```python
from build123d import *

# Parameters (mm, degrees)
F0_W     = 76.2
F0_H     = 50.8
F0_R     = 12.7
F1_DEPTH = 25.4
F2_W     = 6.35
F2_H     = 50.8
F3_DEPTH = 2.54
F5_R     = 10.0587183536
F6_DEPTH = 25.4
F7_DEPTH = 12.446
F8_DEPTH = 70.358


with BuildPart() as f1:
    # F0 (on Top) → F1 (new body)
    with BuildSketch(Plane.XY):
        with Locations((3.2262094319, -2.200336157)):
            Rectangle(F0_W, F0_H)
        Circle(F0_R, mode=Mode.SUBTRACT)
    extrude(amount=F1_DEPTH)

    # F2 (on face) → F3 (cut)
    with BuildSketch(Plane.XY.offset(25.4)):
        with Locations((-29.1587905681, -2.200336157)):
            Rectangle(F2_W, F2_H)
        with BuildLine():
            Line((-6.35, -10.9985226281), (-6.35, -27.600336157))
            Line((-6.35, -27.600336157), (6.35, -27.600336157))
            Line((6.35, -27.600336157), (6.35, -10.9985226281))
            ThreePointArc((6.35, -10.9985226281), (0, -12.7), (-6.35, -10.9985226281))
        make_face()
        with BuildLine():
            Line((6.35, 23.199663843), (-6.35, 23.199663843))
            Line((-6.35, 23.199663843), (-6.35, 10.9985226281))
            ThreePointArc((-6.35, 10.9985226281), (0, 12.7), (6.35, 10.9985226281))
            Line((6.35, 10.9985226281), (6.35, 23.199663843))
        make_face()
    extrude(amount=-F3_DEPTH, mode=Mode.SUBTRACT)

    # F5 (on face) → F6 (join)
    with BuildSketch(Plane.YZ.offset(41.3262094319)):
        with Locations((-2.200336157, 12.7)):
            Circle(F5_R)
    extrude(amount=F6_DEPTH)

    # F5 (on face) → F7 (join)
    with BuildSketch(Plane.YZ.offset(41.3262094319)):
        with Locations((-2.200336157, 12.7)):
            Circle(F5_R)
    extrude(amount=-F7_DEPTH)

    # F4 (on face) → F8 (cut)
    with BuildSketch(Plane.XZ.offset(27.600336157)):
        Polygon((30.2859525938, 25.4), (17.5859525938, 25.4), (14.6530132263, 20.32), (33.2188919613, 20.32), align=None)
    extrude(amount=-F8_DEPTH, mode=Mode.SUBTRACT)


solid = f1.part
```
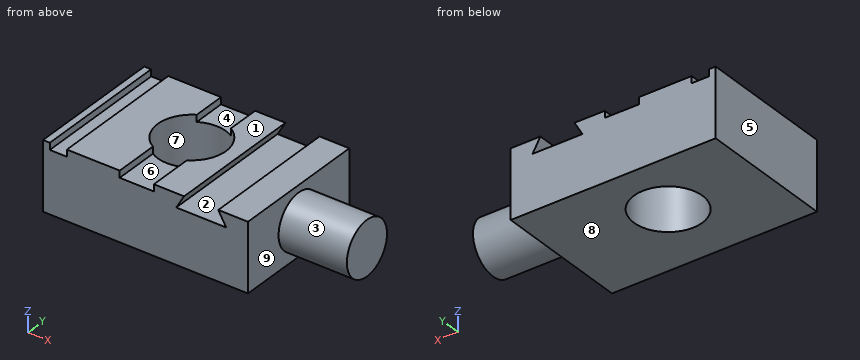
Read the model definition and answer for the solid it produces. Units are mm, in the model's axes. Face numbers are marked on the shaded views. A direction names the side the tool comes from. Give positions to 0.01 mm unless a question says otherwise; leave off trailing zeros. Order: outer loops, then holes, each group sorted by start corner. A loop starts at its lowest first (then second) coordinate and runs counter-clockwise, first axis right, second up. Notation, with made-up numbers: (77, -7) -> (129, -7) arc R18 ccw to (129, 19) -> close; hole circle Ø2 at (62.25, 43.5). An arc over 180 degrees is marked (long way). Write item = value, one per line.
1. A cutting plane is placed at A-A, the plane z = 21.75. Write down the section's boundary in (x, y), and give its area (3 significant figures).
Numbers:
outline = (-34.87, -27.6) -> (15.48, -27.6) -> (15.48, 23.2) -> (-34.87, 23.2) -> close; (32.39, -27.6) -> (41.33, -27.6) -> (41.33, -6.59) -> (66.73, -6.59) -> (66.73, 2.19) -> (41.33, 2.19) -> (41.33, 23.2) -> (32.39, 23.2) -> close; hole circle Ø25.4 at (0, 0)
area = 2,730 mm²
2. Given pin 1 (0.8 mm diameter, centred on y = 4.5, z = 24, fed in from +X); pin 2 (20.5 mm diameter, centred on x = 0, y = 0, fed in from -Z), each flat-ended and moving along its own axis, determine where each tip first touches the part or whether it passes through.
Numbers:
pin_1 = 41.33
pin_2 = through
3. A cutting plane is placed at B-B, the plane x = 0. Write down the section's boundary in (y, z), and give its area (3 significant figures).
Numbers:
outline = (-27.6, 0) -> (-12.7, 0) -> (-12.7, 22.86) -> (-27.6, 22.86) -> close; (12.7, 0) -> (23.2, 0) -> (23.2, 22.86) -> (12.7, 22.86) -> close
area = 581 mm²
4. Straight lines are drawn through the part: line 1 along Y through (x, z) = (0, 15.75); line 2 along X through (y, z) = (0, 18); line 3 along X through (y, z) = (0.5, 21.25). For each, find the intervals that lie inside material, in ascending order.
Numbers:
line_1 = -27.6 to -12.7, 12.7 to 23.2
line_2 = -34.87 to -12.7, 12.7 to 66.73
line_3 = -34.87 to -12.69, 12.69 to 15.19, 32.68 to 66.73
5. A cutting plane is placed at D-D, the plane z = 12.7. Write down the section's boundary in (x, y), and give its area (3 significant figures).
Numbers:
outline = (-34.87, -27.6) -> (41.33, -27.6) -> (41.33, -12.26) -> (66.73, -12.26) -> (66.73, 7.86) -> (41.33, 7.86) -> (41.33, 23.2) -> (-34.87, 23.2) -> close; hole circle Ø25.4 at (0, 0)
area = 3,880 mm²
6. For the marked faces 1, 2, 3, 4 and 5, determine the directions among +Z, -Z, +X, -X, +Y, -Y from which every point of the face is accessible in a straight line to the end or side of a thin tool.
Numbers:
face_1 = +Z, +X, -X, +Y, -Y
face_2 = +Y, -Y
face_3 = +X
face_4 = +Z, +Y, -Y
face_5 = +Z, -Z, -X, +Y, -Y
7. A cutting plane is placed at C-C, the plane y = -5. Write down the section's boundary in (x, z), and give its area (3 significant figures).
Numbers:
outline = (-34.87, 0) -> (-11.67, 0) -> (-11.67, 25.4) -> (-25.98, 25.4) -> (-25.98, 22.86) -> (-32.33, 22.86) -> (-32.33, 25.4) -> (-34.87, 25.4) -> close; (11.67, 0) -> (41.33, 0) -> (41.33, 3.04) -> (66.73, 3.04) -> (66.73, 22.36) -> (41.33, 22.36) -> (41.33, 25.4) -> (30.29, 25.4) -> (33.22, 20.32) -> (14.65, 20.32) -> (17.59, 25.4) -> (11.67, 25.4) -> close
area = 1,740 mm²
8. The mould has two halves that part along X. Classify the marked faces 6, 7, 8 and 9: +X half, -X half, draft (parallel to the pull), parting line (faces both ways), or undercut.
Numbers:
face_6 = undercut
face_7 = undercut
face_8 = draft
face_9 = +X half
